Input: part model. Units: mm. Frame: model coordinates. Round coordinates to 2 decimals unless told otherwise and drop trailing zeros. Loops run counter-clockwise (first coordinate to the right, second up) from the corner with the lowest first, then second, coordinate; pieces in that order, holes last. Notation, with made-up numbers: M 25.5,61 L 44.5,61 A9 cw 44.5,75 Z; hole C 67,5.25 d4. An arc over 180 degrees is marked long. Return JSON: item names as keys, results as strings. Group by question number.
1) Section C-C (z = 3). Output: boundary loops of the cut face in (x, y).
2) Contact query for flat-ended pins moving along their axis: P1, Ø2.5, axis at x = 23.69, y = -23.69, coming from the -Z side; P2, Ø4, axis at x = -7, z = 5, coming from the -Y side; P3, Ø1.2, axis at x = 32.36, y = -8.67, coming from the -Z side (3 decimals); P4, Ø2, axis at y = 3, z = 3, coming from the +X side. Output: stop coordinate, or through.
3) Mould query, pull axis Y, two halves, no side actions, for faces 1 (the face through (-30.928, -14.993, 5.603)), 2 (the face through (8.7, 28.3, 5.4)). Classes: +Y half, -Y half, draft (parallel to the pull), parting line (faces both ways), or undercut.
4) Material intervals for line 1 (Y direction, x = 0, z = 3.9); line 2 (X direction, y = 1, z = 4.5); line 3 (Y direction, x = 29.5, z = 5.75), sorted ascending. Write a range as from..to.
5) Section A-A (x = 0). Output: boundary loops of the cut face in (y, z), plus the area to 3 significant figures.
from build123d import *

# Parameters (mm, degrees)
SKETCH2_R          = 2.6
SKETCH2_R_2        = 1
CUT_EXTRUDE1_DEPTH = 55.614650049
CIRPATTERN1_COUNT  = 12


with BuildPart() as part:
    # Sketch1 → Revolve-Thin1 (revolve)
    with BuildSketch(Plane(origin=(0, 0, 0), x_dir=(0, 0, -1), z_dir=(1, 0, 0)), mode=Mode.PRIVATE) as revolve_thin1_sk:
        Polygon((0, 29), (-5.8, 29), (-5.8, 38), (-8, 38), (-8, 38.4), (-5.4, 38.4), (-5.4, 29.4), (0, 29.4), align=None)
    revolve(revolve_thin1_sk.sketch.rotate(Axis((0, 0, 0), (0, 0, 1)), 90), axis=Axis((0, 0, 0), (0, 0, 1)))

    # Sketch2 → Cut-Extrude1 (cut, through all)
    with BuildSketch(Plane.XY.offset(5.8)):
        with Locations((0, 33.5)):
            Circle(SKETCH2_R)
        with Locations((-8.670438011, 32.358515181)):
            Circle(SKETCH2_R_2)
    cut_extrude1 = extrude(amount=-CUT_EXTRUDE1_DEPTH, mode=Mode.SUBTRACT)

    # CirPattern1: Cut-Extrude1 ×12 about axis
    cirpattern1_axis = Axis((0, 0, 0), (0, 0, 1))
    for i in range(1, CIRPATTERN1_COUNT):
        add(cut_extrude1.rotate(cirpattern1_axis, i * 360 / CIRPATTERN1_COUNT), mode=Mode.SUBTRACT)


solid = part.part
Returned:
{
 "1": {"outline": "C 0,0 d58.8; hole C 0,0 d58"},
 "2": {"P1": "stops at z = 5.4", "P2": "stops at y = -38.07", "P3": "passes through", "P4": "stops at x = 29.33"},
 "3": {"face 1": "undercut", "face 2": "draft"},
 "4": {"line 1": "y = -29.4..-29, 29..29.4", "line 2": "x = -29.38..-28.98, 28.98..29.38", "line 3": "y = -24.58..-19.3, -14.2..14.2, 19.3..24.58"},
 "5": {"outline": "M -38.4,5.4 L -36.1,5.4 L -36.1,5.8 L -38,5.8 L -38,8 L -38.4,8 Z; M -30.9,5.4 L -29.4,5.4 L -29.4,0 L -29,0 L -29,5.8 L -30.9,5.8 Z; M 29,0 L 29.4,0 L 29.4,5.4 L 30.9,5.4 L 30.9,5.8 L 29,5.8 Z; M 36.1,5.4 L 38.4,5.4 L 38.4,8 L 38,8 L 38,5.8 L 36.1,5.8 Z", "area": "9.44 mm^2"}
}
